Could you check a few things on this model? Use its own coordinates, in mm. Face numbers are marked on the shaded views. Give positions to 0.01 mm unless a question says otherwise; leave off trailing zeros. Loops run counter-clockwise (first coordinate to the right, second up) from the corner with the lowest first, then second, coordinate; pieces in that order, holes last. Notation, with made-up numbers: (-40, 45.5) -> (-7, 45.5) arc R4 cw to (-7, 49.5) -> close; hole circle Ø3 at (44.5, 20). An arc over 180 degrees is marked (long way). Write item = value, one per line. Start each with the question number.
1) I want a section at A-A (z = 2.25). List the corners of the cut face in (x, y) for me.
2) I'm going to push flat-ended pins straight in: pin 1 Ø1.5 at (x, y) = (-1.5, 0) entering from -Z; pin 2 Ø0.8 at (x, y) = (1, 2.5) entering from +Z. Where does each tip first touch, or does it pass through?
3) I need wall thicknesses on probe 1 along X at (y, z) = (1.3, 2); probe 2 along Z at (x, y) = (0, 1.65); probe 3 along Y at (x, z) = (0.75, -3.5). Which ranges of each line are inside material? Lowest first, please. Write a range as from..to.
4) I want a section at B-B (z = -0.5). List the corners of the cut face in (x, y) for me.
5) If we mould it in two halves opening along X, with no side actions, what happens to the marked faces 1, 2 and 3? For each: +X half, -X half, draft (parallel to the pull), parting line (faces both ways), or undercut.
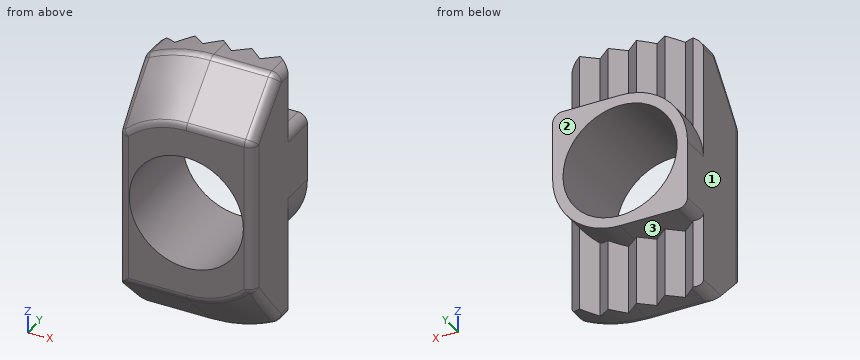
from build123d import *

# Parameters (mm, degrees)
SKETCH1_W                        = 5.7
SKETCH1_H                        = 11.5
BOSS_EXTRUDE1_DEPTH              = 1.35
BOSS_EXTRUDE2_DEPTH              = 11.5
BOSS_EXTRUDE4_DEPTH              = 1.5
CUT_EXTRUDE3_DEPTH               = 3.5
CHAMFER2_SIZE                    = 2
F_10_32_TAPPED_HOLE3_D           = 4.0386
F_10_32_TAPPED_HOLE3_DEPTH       = 12.02944
F_10_32_TAPPED_HOLE3_CBORE_D     = 4.826
F_10_32_TAPPED_HOLE3_CBORE_DEPTH = 9.652
F_10_32_TAPPED_HOLE3_TIP         = 1.213317848
FILLET2_R                        = 0.4


with BuildPart() as part:
    # Sketch1 → Boss-Extrude1 (new, symmetric)
    with BuildSketch(Plane(origin=(0, 0, 0), x_dir=(1, 0, 0), z_dir=(0, 1, 0))):
        Rectangle(SKETCH1_W, SKETCH1_H)
    extrude(amount=BOSS_EXTRUDE1_DEPTH, both=True)

    # Sketch2 → Boss-Extrude2 (add)
    with BuildSketch(Plane.XY.offset(5.75)):
        Polygon((-2.85, 1.35), (-1.95, 1.35), (-2.55, 1.85), (-2.85, 1.6), align=None)
        Polygon((-1.95, 1.35), (-0.75, 1.35), (-1.35, 1.85), align=None)
        Polygon((-0.75, 1.35), (0.45, 1.35), (-0.15, 1.85), align=None)
        Polygon((0.45, 1.35), (1.65, 1.35), (1.05, 1.85), align=None)
        Polygon((2.85, 1.35), (2.25, 1.85), (1.65, 1.35), align=None)
    extrude(amount=-BOSS_EXTRUDE2_DEPTH)

    # Sketch7 → Boss-Extrude4 (add)
    with BuildSketch(Plane.XZ.offset(-1.35)):
        with BuildLine():
            Line((0, 2.85), (2.45, 2.85))
            ThreePointArc((2.45, 2.85), (2.732842712, 2.732842712), (2.85, 2.45))
            Line((2.85, 2.45), (2.85, 0))
            ThreePointArc((2.85, 0), (2.015254326, -2.015254326), (0, -2.85))
            Line((0, -2.85), (-2.45, -2.85))
            ThreePointArc((-2.45, -2.85), (-2.732842712, -2.732842712), (-2.85, -2.45))
            Line((-2.85, -2.45), (-2.85, 0))
            ThreePointArc((-2.85, 0), (-2.015254326, 2.015254326), (0, 2.85))
        make_face()
    extrude(amount=-BOSS_EXTRUDE4_DEPTH)

    # Sketch8 → Cut-Extrude3 (cut)
    with BuildSketch(Plane.XZ.offset(1.35)):
        with BuildLine():
            Line((-2.85, 4.993996396), (-2.85, 5.75))
            Line((-2.85, 5.75), (0, 5.75))
            ThreePointArc((0, 5.75), (-1.474282999, 5.557786397), (-2.85, 4.993996396))
        make_face()
        with BuildLine():
            Line((0, -5.75), (2.85, -5.75))
            Line((2.85, -5.75), (2.85, -4.993996396))
            ThreePointArc((2.85, -4.993996396), (1.474282999, -5.557786397), (0, -5.75))
        make_face()
    extrude(amount=-CUT_EXTRUDE3_DEPTH, mode=Mode.SUBTRACT)

    # Chamfer2
    chamfer2_edges = [part.edges().sort_by_distance(p)[0] for p in [
        (1.425, -1.35, 5.75),
        (-1.474282999, -1.35, 5.557786397),
        (-1.425, -1.35, -5.75),
        (1.474282999, -1.35, -5.557786397),
    ]]
    chamfer(chamfer2_edges, length=CHAMFER2_SIZE)

    # #10-32 Tapped Hole3
    with Locations(Plane.XZ.offset(1.35)):
        with Locations((0, 0)):
            CounterBoreHole(F_10_32_TAPPED_HOLE3_D / 2, F_10_32_TAPPED_HOLE3_CBORE_D / 2, F_10_32_TAPPED_HOLE3_CBORE_DEPTH, depth=F_10_32_TAPPED_HOLE3_DEPTH)
            with Locations((0, 0, -(F_10_32_TAPPED_HOLE3_DEPTH + F_10_32_TAPPED_HOLE3_TIP / 2))):  # 118° drill point
                Cone(0, F_10_32_TAPPED_HOLE3_D / 2, F_10_32_TAPPED_HOLE3_TIP, mode=Mode.SUBTRACT)

    # Fillet2
    fillet2_edges = [part.edges().sort_by_distance(p)[0] for p in [
        (1.425, 0.65, 5.75),
        (1.425, -1.35, 3.75),
        (-1.425, 0.65, -5.75),
        (-1.425, -1.35, -3.75),
        (-1.474282999, 0.65, 5.557786397),
        (-1.568909939, -1.35, 3.406027246),
        (-2.85, -0.391617372, 3.747848312),
        (1.474282999, 0.65, -5.557786397),
        (1.568909939, -1.35, -3.406027246),
        (2.85, -0.391617372, -3.747848312),
        (2.85, 1, 5.75),
        (2.85, -0.35, 4.75),
        (-2.85, 1.125, 4.993996396),
        (-2.85, -1.35, -0.656394239),
        (-2.85, 1.125, -5.75),
        (2.85, -1.35, 0.656394239),
        (2.85, 1, -4.993996396),
    ]]
    fillet(fillet2_edges, radius=FILLET2_R)


solid = part.part
Answer list:
q1.outline = (-2.85, -0.95) arc R0.4 ccw to (-2.45, -1.35) -> (-0.87, -1.35) -> (-0.87, 2.85) -> (-1.75, 2.85) -> (-1.75, 1.52) -> (-1.95, 1.35) -> (-2.55, 1.85) -> (-2.85, 1.6) -> close; (0.87, -1.35) -> (2.45, -1.35) arc R0.4 ccw to (2.85, -0.95) -> (2.85, 2.85) -> (0.87, 2.85) -> close
q2.pin_1 = -5.74
q2.pin_2 = 2.85
q3.probe_1 = -2.85..-1.35, 1.35..2.85
q3.probe_2 = -5.75..-2.41, 2.41..5.75
q3.probe_3 = -1.35..1.6
q4.outline = (-2.85, -0.95) arc R0.4 ccw to (-2.45, -1.35) -> (-2.36, -1.35) -> (-2.36, 2.85) -> (-2.85, 2.85) -> close; (2.36, -1.35) -> (2.45, -1.35) arc R0.4 ccw to (2.85, -0.95) -> (2.85, 1.35) -> (2.81, 1.39) -> (2.81, 2.85) -> (2.36, 2.85) -> close
q5.face_1 = -X half
q5.face_2 = draft
q5.face_3 = undercut
